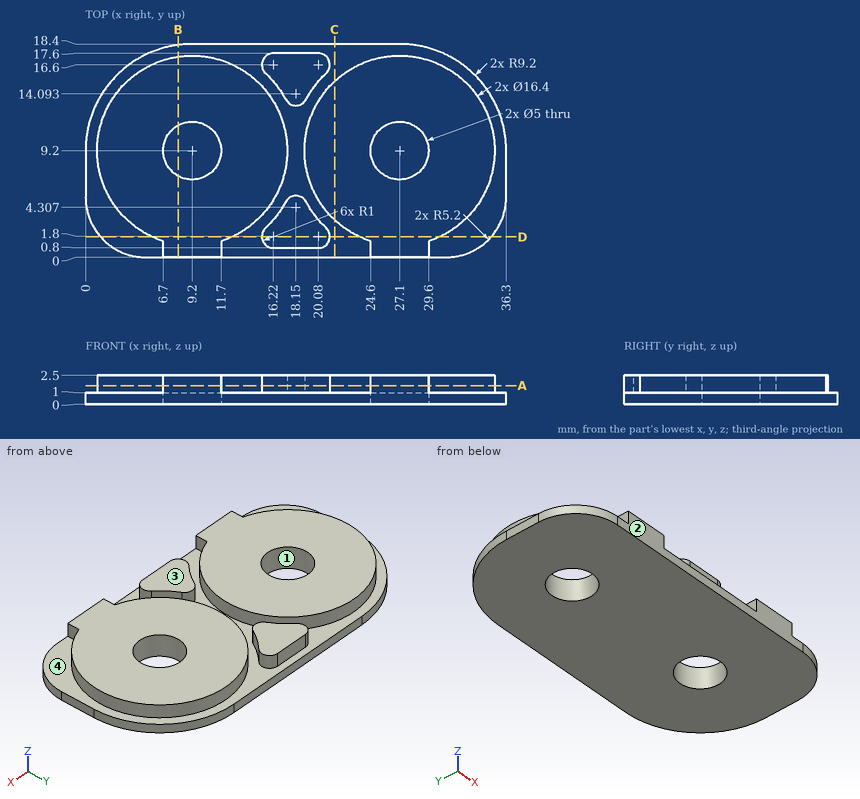
Design review of the part shown in the three views and the two pictorial views. Dimensions are in mm from the part's minimum x, y and z. A direction names the side the tool comes from. Give positions to 0.01 mm unless a question says otherwise; leave off trailing zeros. Loops run counter-clockwise (first coordinate to the right, second up) from the corner with the lowest first, then second, coordinate; pieces in that order, holes last. Notation, with made-up numbers: M 38.5,52.25 L 82.5,52.25 A28 cw 82.5,74.25 Z; hole C -20.75,60 d2. An arc over 180 degrees is marked long. Write item = value, one per line.
Q1. We need section C-C (x = 21.5). Give the boundary of the cut face in (y, z).
Output values:
outline = M 0,0 L 18.4,0 L 18.4,1 L 15.19,1 L 15.19,2.5 L 3.21,2.5 L 3.21,1 L 0,1 Z
Q2. We need section D-D (y = 1.75). Give the boundary of the cut face in (x, z).
Output values:
outline = M 1.31,0 L 34.99,0 L 34.99,1 L 30.53,1 L 30.53,2.5 L 23.67,2.5 L 23.67,1 L 21.08,1 L 21.08,2.5 L 15.22,2.5 L 15.22,1 L 12.63,1 L 12.63,2.5 L 5.77,2.5 L 5.77,1 L 1.31,1 Z
Q3. For the marked faces 3 and 4, list the 3-axis set-ups (+Z, -Z, +X, -X, +Y, -Y) from which the entire face can be reached by the end or side of a thin tool; tool diameter is ignored.
Output values:
face_3 = +Z, +X, -X, +Y, -Y
face_4 = +Z
Q4. We need section B-B (x = 8). Give the boundary of the cut face in (y, z).
Output values:
outline = M 0,0 L 7.01,0 L 7.01,2.5 L 0,2.5 Z; M 11.39,0 L 18.32,0 L 18.32,1 L 17.31,1 L 17.31,2.5 L 11.39,2.5 Z
Q5. We need section A-A (z = 1.6). Count the separate pieces of the cut face and the enclosed holes in it, plus the area to 3 significant figures.
Output values:
separate_pieces = 4
enclosed_holes = 2
area = 430 mm^2
Q6. Draft analysis for pull direction X (two halves, no side actions). For the marked faces 1 and 2, state which applies: +X half, -X half, draft (parallel to the pull), parting line (faces both ways), or undercut.
Output values:
face_1 = undercut
face_2 = draft
Q7. Insertion check: pin 1 (4.5 mm diameter, centred on x = 27.1, y = 9.2, fed in from -Z); pin 2 (0.8 mm diameter, centred on x = 19, z = 2, fed in from -Y); pin 3 (5 mm diameter, centred on x = 28, y = 14, fed in from -Z); pin 4 (1.5 mm diameter, centred on y = 1, z = 2, fed in from -X) (1 decimal). Each pin has a flat end and moves straight along its axis. Give the tip position at first contact, or say it passes through.
Output values:
pin_1 = through
pin_2 = 0.8
pin_3 = 0
pin_4 = 5.8
Q8. To check wall thickness, follow line 1 (X direction, y = 13.5, z = 2.3) (1 decimal); line 2 (Y direction, x = 27.1, z = 0.95); line 3 (Y direction, x = 27.1, z = 1.6). State the ranges of each line that lie inside material, in increasing order. Write a range as [from, to].
Output values:
line_1 = [2.2, 16.2], [17.3, 19], [20.1, 34.1]
line_2 = [0, 6.7], [11.7, 18.4]
line_3 = [0, 6.7], [11.7, 17.4]
